Work out the finished part from the listing and answer in its coordinate system (mm). A direction names the side the tool comes from. Give positions to 0.01 mm unless a question says otherwise; leave off trailing zeros. Write each loop counter-clockwise with the first axis right and the second up, starting at its lowest first coordinate (ties: lowest second). Pieces come first, ordered by that corner, then holes. Notation, with made-up numbers: (35.5, -1) - (63.5, -1) arc R21 ccw to (63.5, 6) - close; hole circle Ø3 at (33, 88). An arc over 180 degrees is marked (long way). Write item = value, one per line.
from build123d import *


with BuildPart() as part:
    # Croquis1 → Revolución1 (revolve)
    with BuildSketch(Plane(origin=(0, 0, 0), x_dir=(1, 0, 0), z_dir=(0, 1, 0))):
        with BuildLine():
            Line((-0.88053939, 16), (-5, 16))
            ThreePointArc((-5, 16), (-5.707106781, 15.707106781), (-6, 15))
            Line((-6, 15), (-6, 11.50146596))
            Line((-6, 11.50146596), (-5, 11.50146596))
            Line((-5, 11.50146596), (-5, 15))
            Line((-5, 15), (0, 15))
            Line((0, 15), (0, 16.5))
            Line((0, 16.5), (0.055870191, 16.649091044))
            ThreePointArc((0.055870191, 16.649091044), (-0.310850421, 16.178139624), (-0.88053939, 16))
        make_face()
    revolve(axis=Axis((0, 0, 0), (-1, 0, 0)))


solid = part.part
1. Given pin 1 (1.5 mm diameter, centred on x = -2.5, z = -4, fed in from +Y); pin 2 (1 mm diameter, centred on x = -5, y = 2, fed in from +Z); pin 3 (2 mm diameter, centred on x = -5, z = -12, fed in from +Y), each flat-ended and moving along its own axis, determine where each tip first touches the part or whether it passes through.
Solution:
pin_1 = 15.67
pin_2 = 15.93
pin_3 = 11.62
2. Find section C-C, the plane x = -2. Give the vertices of the cut face in (y, z).
Solution:
outline = circle Ø32 at (0, 0); hole circle Ø30 at (0, 0)
3. Straight lines are drawn through the part: line 1 (Z direction, x = -2, y = 0); line 2 (Y direction, x = -2.25, z = 5). For each, find the intervals that lie inside material, in ascending order.
Solution:
line_1 = -16 to -15, 15 to 16
line_2 = -15.2 to -14.14, 14.14 to 15.2
4. Find section A-A, the plane y = 0. Give the vertices of the cut face in (x, z).
Solution:
outline = (-6, -15) arc R1 ccw to (-5, -16) - (-0.88, -16) arc R1 cw to (0.06, -16.65) - (0, -16.5) - (0, -15) - (-5, -15) - (-5, -11.5) - (-6, -11.5) - close; (-6, 11.5) - (-5, 11.5) - (-5, 15) - (0, 15) - (0, 16.5) - (0.06, 16.65) arc R1 cw to (-0.88, 16) - (-5, 16) arc R1 ccw to (-6, 15) - close
5. A tool of negligible diameter and unlimited length cuts with its end or side. For faces 1 (the flat face through (0, 15, 4)), 2 (the cylindrical face through (-5.49, 11.23, 2.49)), from which of +Z, -Z, +X, -X, +Y, -Y can it reach the whole face along a straight path? Write none if from no direction.
Solution:
face_1 = +X
face_2 = +X, -X
6. For a pull along Y with two mould halves and no side action, classify faces 3 (the flat face through (-5, 9, 8)), 4 (the flat face through (-6, 9, -8)), 5 (the cylindrical face through (-2.97, 15.62, 3.47)) as pulls with the +Y half, pulls with the -Y half, needs draft (parallel to the pull), parting line crosses it, or undercut.
Solution:
face_3 = undercut
face_4 = needs draft
face_5 = parting line crosses it
